```python
from build123d import *

# Parameters (mm, degrees)
SKETCH1_W               = 18.034
SKETCH1_H               = 22.7965
SKETCH1_W_2             = 15.748
SKETCH1_H_2             = 9.652
BOSS_EXTRUDE1_DEPTH     = 5.9055
SKETCH2_W               = 1.27
SKETCH2_H               = 1.016
SKETCH2_H_2             = 1.4605
CUT_EXTRUDE_THIN2_DEPTH = 3.175
CHAMFER1_SIZE           = 0.254
CHAMFER2_SIZE           = 0.508
FILLET1_R               = 0.762
F_0_80_TAPPED_HOLE1_D   = 1.19126


with BuildPart() as part:
    # Sketch1 → Boss-Extrude1 (new body)
    with BuildSketch(Plane.XY):
        with Locations((22.86, -68.54825)):
            Rectangle(SKETCH1_W, SKETCH1_H)
        with Locations((22.86, -62.992)):
            Rectangle(SKETCH1_W_2, SKETCH1_H_2, mode=Mode.SUBTRACT)
        with Locations((22.86, -74.1045)):
            Rectangle(SKETCH1_W_2, SKETCH1_H_2, mode=Mode.SUBTRACT)
    extrude(amount=BOSS_EXTRUDE1_DEPTH)

    # Sketch2 → Cut-Extrude-Thin2 (cut)
    with BuildSketch(Plane(origin=(0, 0, 0), x_dir=(-1, 0, 0), z_dir=(0, 0, -1))):
        with Locations((-22.86, -79.4385)):
            Rectangle(SKETCH2_W, SKETCH2_H)
        with Locations((-19.177, -57.658)):
            Rectangle(SKETCH2_W, SKETCH2_H)
        with Locations((-26.543, -57.658)):
            Rectangle(SKETCH2_W, SKETCH2_H)
        with Locations((-22.86, -68.54825)):
            Rectangle(SKETCH2_W, SKETCH2_H_2)
        with Locations((-19.177, -68.54825)):
            Rectangle(SKETCH2_W, SKETCH2_H_2)
        with Locations((-26.543, -68.54825)):
            Rectangle(SKETCH2_W, SKETCH2_H_2)
    extrude(amount=-CUT_EXTRUDE_THIN2_DEPTH, mode=Mode.SUBTRACT)

    # Chamfer1
    chamfer1_edges = [part.edges().sort_by_distance(p)[0] for p in [
        (22.225, -68.54825, 3.175),
        (23.495, -68.54825, 3.175),
        (25.908, -68.54825, 3.175),
        (27.178, -68.54825, 3.175),
        (23.495, -79.4385, 3.175),
        (22.225, -79.4385, 3.175),
        (19.812, -57.658, 3.175),
        (18.542, -57.658, 3.175),
        (27.178, -57.658, 3.175),
        (25.908, -57.658, 3.175),
        (18.542, -68.54825, 3.175),
        (19.812, -68.54825, 3.175),
    ]]
    chamfer(chamfer1_edges, length=CHAMFER1_SIZE)

    # Chamfer2
    chamfer2_edges = [part.edges().sort_by_distance(p)[0] for p in [
        (31.877, -57.15, 2.95275),
        (31.877, -79.9465, 2.95275),
        (13.843, -79.9465, 2.95275),
        (13.843, -57.15, 2.95275),
    ]]
    chamfer(chamfer2_edges, length=CHAMFER2_SIZE)

    # Fillet1
    fillet1_edges = [part.edges().sort_by_distance(p)[0] for p in [
        (30.734, -67.818, 2.95275),
        (30.734, -58.166, 2.95275),
        (14.986, -78.9305, 2.95275),
        (30.734, -78.9305, 2.95275),
        (14.986, -58.166, 2.95275),
        (14.986, -67.818, 2.95275),
        (30.734, -69.2785, 2.95275),
        (14.986, -69.2785, 2.95275),
    ]]
    fillet(fillet1_edges, radius=FILLET1_R)

    # #0-80 Tapped Hole1 (through all)
    with Locations(Plane(origin=(0, 0, 0), x_dir=(-1, 0, 0), z_dir=(0, 0, -1))):
        with Locations((-30.9245, -68.54825), (-14.7955, -68.54825)):
            Hole(F_0_80_TAPPED_HOLE1_D / 2)


solid = part.part
```
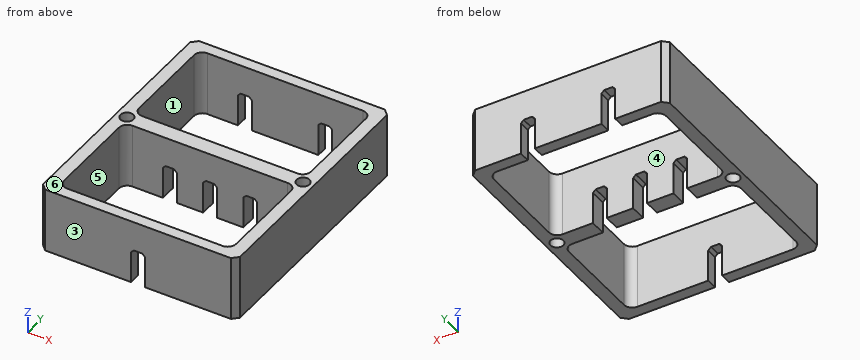
Can you work these out from the model? Positions are in its coordinate system, mm. Face numbers are marked on the shaded views. A direction names the side the tool comes from. Coordinates: 2 decimals unless noted, no trailing zeros. Order: outer loops, then holes, each group sorted by start corner. A loop starts at its lowest first (then second) coordinate and runs counter-clockwise, first axis right, second up. Notation, with made-up numbers: (82.25, 26.5) - (96.25, 26.5) arc R7 ccw to (96.25, 38.5) - close; hole circle Ø6 at (19.25, 36). An arc over 180 degrees is marked (long way). Answer in a Markdown table with one row per item.
1. If I drill on line 1 along Y through (x, z) = (18.75, 5.05); line 2 along X through (y, z) = (-66.75, 2.8); line 3 along Y through (x, z) = (30.5, 2.6), over which ranges is the centre line in solid material (lowest first)?
Reply:
| item | result |
|---|---|
| line 1 | y = -79.95 to -78.93, -69.28 to -67.82, -58.17 to -57.15 |
| line 2 | x = 13.84 to 14.99, 30.73 to 31.88 |
| line 3 | y = -79.95 to -78.72, -69.49 to -68.97, -68.13 to -67.61, -58.38 to -57.15 |
2. Suppose I cut it at C-C (z = 5). Please give me the cut outline in (x, y), and give its area (3 significant figures).
Reply:
| item | result |
|---|---|
| outline | (13.84, -79.44) - (14.35, -79.95) - (31.37, -79.95) - (31.88, -79.44) - (31.88, -57.66) - (31.37, -57.15) - (14.35, -57.15) - (13.84, -57.66) - close; hole circle Ø1.19 at (14.8, -68.55); hole (14.99, -78.17) arc R0.76 ccw to (15.75, -78.93) - (29.97, -78.93) arc R0.76 ccw to (30.73, -78.17) - (30.73, -70.04) arc R0.76 ccw to (29.97, -69.28) - (15.75, -69.28) arc R0.76 ccw to (14.99, -70.04) - close; hole (14.99, -67.06) arc R0.76 ccw to (15.75, -67.82) - (29.97, -67.82) arc R0.76 ccw to (30.73, -67.06) - (30.73, -58.93) arc R0.76 ccw to (29.97, -58.17) - (15.75, -58.17) arc R0.76 ccw to (14.99, -58.93) - close; hole circle Ø1.19 at (30.92, -68.55) |
| area | 105 mm^2 |
3. Suppose I cut it at D-D (x = 17). Please give me the cut outline in (y, z), and give its area (3 significant figures).
Reply:
| item | result |
|---|---|
| outline | (-79.95, 0) - (-78.93, 0) - (-78.93, 5.91) - (-79.95, 5.91) - close; (-69.28, 0) - (-67.82, 0) - (-67.82, 5.91) - (-69.28, 5.91) - close; (-58.17, 0) - (-57.15, 0) - (-57.15, 5.91) - (-58.17, 5.91) - close |
| area | 20.6 mm^2 |
4. For the marked faces 5 and 6, which set-ups out of +Z, -Z, +X, -X, +Y, -Y let a thin tool reach every point of the face, with its end or its side?
Reply:
| item | result |
|---|---|
| face 5 | +Z, -Z |
| face 6 | +Z, +X, -X, +Y, -Y |
5. Suppose I cut it at A-A (x = 19.25). Give the number of separate pieces and of enclosed holes in the cut face, and give its area (3 significant figures).
Reply:
| item | result |
|---|---|
| separate pieces | 3 |
| enclosed holes | 0 |
| area | 12.8 mm^2 |
6. If we mould it in two halves opening along Y, with no side actions, what happens to the marked faces 1, 2, 3 and 4? For each: pulls with the +Y half, pulls with the -Y half, needs draft (parallel to the pull), parting line crosses it, or undercut.
Reply:
| item | result |
|---|---|
| face 1 | undercut |
| face 2 | needs draft |
| face 3 | pulls with the -Y half |
| face 4 | undercut |
7. Suppose I cut it at B-B (y = -62). Please give me the cut outline in (x, z), and give its area (3 significant figures).
Reply:
| item | result |
|---|---|
| outline | (13.84, 0) - (14.99, 0) - (14.99, 5.91) - (13.84, 5.91) - close; (30.73, 0) - (31.88, 0) - (31.88, 5.91) - (30.73, 5.91) - close |
| area | 13.5 mm^2 |
8. For pin 1 (0.8 mm diameter, centred on x = 19, y = -68.5, fed in from -Z); pin 2 (5 mm diameter, centred on x = 26.5, y = -63, fed in from -Z), each with a flat end and sliding along its axis, tell me the tip position at first contact or that it passes through.
Reply:
| item | result |
|---|---|
| pin 1 | stops at z = 2.98 |
| pin 2 | passes through |
